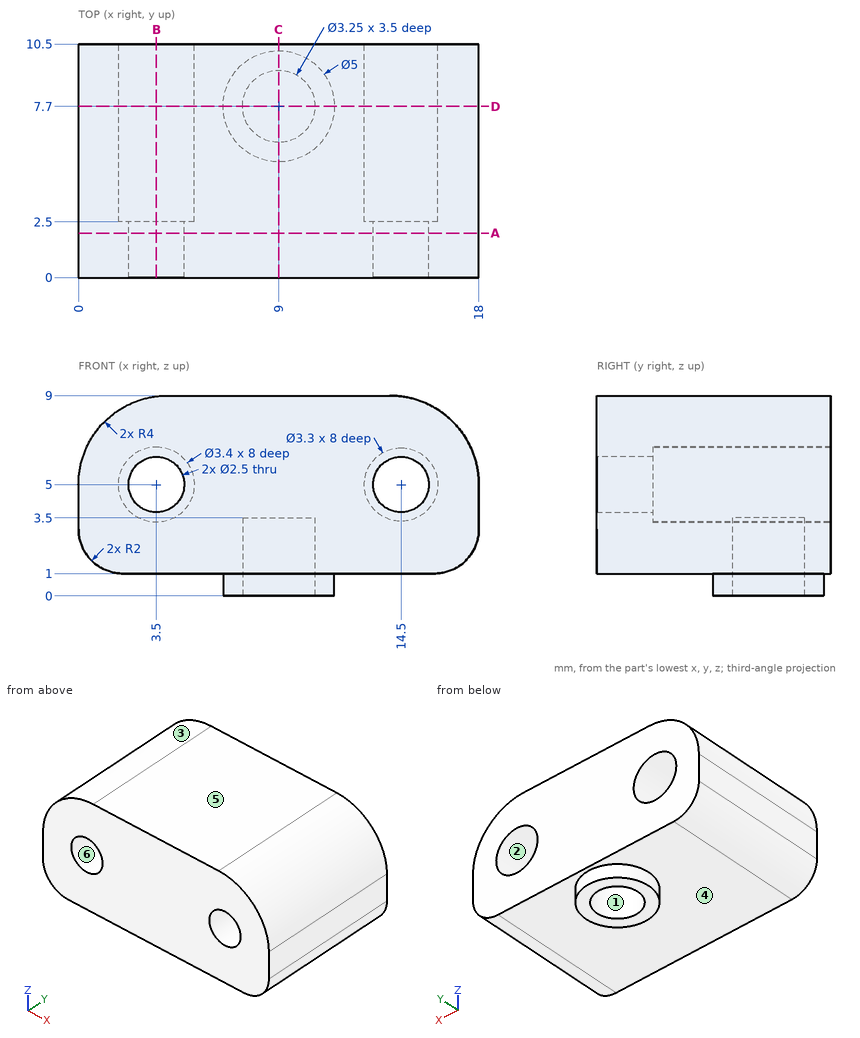
Drawing for the job (mm, zero at the part's lowest x, y, z). A direction names the side the tool comes from. Coordinates: 2 decimals unless noted, no trailing zeros. Order: outer loops, then holes, each group sorted by start corner. A loop starts at its lowest first (then second) coordinate and runs counter-clockwise, first axis right, second up. Notation, with made-up numbers: (69, 52.5) -> (99, 52.5) arc R18 cw to (99, 67.5) -> close; hole circle Ø10 at (-11, 35). An arc over 180 degrees is marked (long way). Answer in a Markdown table with one row per item.
1) Which spindle directions (+Z, -Z, +X, -X, +Y, -Y) get a long thin tool onto all of the face, cutting with end or side? Do the marked faces 1, 2 and 3. Say none if no direction does.
Check values:
| item | result |
|---|---|
| face 1 | -Z |
| face 2 | +Y |
| face 3 | +Z, -X, +Y, -Y |
2) Band-saw the part on D-D (y = 7.7). List the corners of the cut face in (x, z) (3 decimals), and give its area (3 significant figures).
Check values:
| item | result |
|---|---|
| outline | (0, 3) arc R2 ccw to (2, 1) -> (6.5, 1) -> (6.5, 0) -> (7.375, 0) -> (7.375, 3.5) -> (10.625, 3.5) -> (10.625, 0) -> (11.5, 0) -> (11.5, 1) -> (16, 1) arc R2 ccw to (18, 3) -> (18, 5) arc R4 ccw to (14, 9) -> (4, 9) arc R4 ccw to (0, 5) -> close; hole circle Ø3.4 at (3.5, 5); hole circle Ø3.3 at (14.5, 5) |
| area | 111 mm2 |
3) Drill centre lines: line 1 (X direction, y = 0.8, z = 5); line 2 (X direction, y = 8.5, z = 5); line 3 (Z direction, x = 7.75, y = 7.5). Where is each one in solid material? Low to high.
Check values:
| item | result |
|---|---|
| line 1 | 0 to 2.25, 4.75 to 13.25, 15.75 to 18 |
| line 2 | 0 to 1.8, 5.2 to 12.85, 16.15 to 18 |
| line 3 | 3.5 to 9 |
4) Band-saw the part on A-A (y = 2). List the corners of the cut face in (x, z).
Check values:
| item | result |
|---|---|
| outline | (0, 3) arc R2 ccw to (2, 1) -> (16, 1) arc R2 ccw to (18, 3) -> (18, 5) arc R4 ccw to (14, 9) -> (4, 9) arc R4 ccw to (0, 5) -> close; hole circle Ø2.5 at (3.5, 5); hole circle Ø2.5 at (14.5, 5) |
5) Flat gauge pins, fed straight in: P1, Ø3, axis at x = 3.5, z = 5, coming from the -Y side; P2, Ø3, axis at x = 14.5, z = 5, coming from the +Y side; P3, Ø1.5, axis at x = 4, y = 1.5, coming from the -Z side; P4, Ø2.5, axis at x = 9, y = 7.7, coming from the -Z side. Where does each tip first touch, or does it go through?
Check values:
| item | result |
|---|---|
| P1 | y = 0 |
| P2 | y = 2.5 |
| P3 | z = 1 |
| P4 | z = 3.5 |
6) Band-saw the part on C-C (x = 9). List the corners of the cut face in (y, z) (3 decimals), and give its area (3 significant figures).
Check values:
| item | result |
|---|---|
| outline | (0, 1) -> (5.2, 1) -> (5.2, 0) -> (6.075, 0) -> (6.075, 3.5) -> (9.325, 3.5) -> (9.325, 0) -> (10.2, 0) -> (10.2, 1) -> (10.5, 1) -> (10.5, 9) -> (0, 9) -> close |
| area | 77.6 mm2 |
7) Mould opens along Z. For the marked faces 4, 5 and 6 say: pulls with the +Z half, pulls with the -Z half, needs draft (parallel to the pull), parting line crosses it, or undercut.
Check values:
| item | result |
|---|---|
| face 4 | pulls with the -Z half |
| face 5 | pulls with the +Z half |
| face 6 | undercut |
8) Band-saw the part on B-B (x = 3.5). List the corners of the cut face in (y, z), and give its area (3 significant figures).
Check values:
| item | result |
|---|---|
| outline | (0, 1) -> (10.5, 1) -> (10.5, 3.3) -> (2.5, 3.3) -> (2.5, 3.75) -> (0, 3.75) -> close; (0, 6.25) -> (2.5, 6.25) -> (2.5, 6.7) -> (10.5, 6.7) -> (10.5, 8.97) -> (0, 8.97) -> close |
| area | 50.2 mm2 |
